Verification items for the finished model (mm, model axes). A direction names the side the tool comes from. Round coordinates to 2 decimals unless told otherwise and drop trailing zeros. Write each loop counter-clockwise with the first axis right and the second up, starting at its lowest first coordinate (ties: lowest second). Pieces come first, ordered by that corner, then holes. Notation, with made-up numbers: (-28, 26) - (-12, 26) arc R24 cw to (-12, 50) - close; hole circle Ø6 at (22, 5.25). An arc over 180 degrees is marked (long way). Answer as a JSON object with one key per item and string values.
```python
from build123d import *

# Parameters (mm, degrees)
SKETCH032_W     = 42
SKETCH032_H     = 42
PAD111_DEPTH    = 2
SKETCH165_W     = 24
SKETCH165_H     = 24
POCKET008_DEPTH = 1
SKETCH167_W     = 42
SKETCH167_H     = 42
SKETCH167_W_2   = 28
SKETCH167_H_2   = 28
POCKET009_DEPTH = 1
SKETCH300_R     = 1.1
POCKET045_DEPTH = 5


with BuildPart() as part:
    # Sketch032 → Pad111 (new body)
    with BuildSketch(Plane.XZ):
        Rectangle(SKETCH032_W, SKETCH032_H)
    extrude(amount=PAD111_DEPTH)

    # Sketch165 (on Face5 of Pad111) → Pocket008 (cut)
    with BuildSketch(Plane(origin=(0, 0, 0), x_dir=(1, 0, 0), z_dir=(0, 1, 0))):
        Rectangle(SKETCH165_W, SKETCH165_H)
    extrude(amount=-POCKET008_DEPTH, mode=Mode.SUBTRACT)

    # Sketch167 (on Face5 of Pocket008) → Pocket009 (cut)
    with BuildSketch(Plane.XZ.offset(2)):
        Rectangle(SKETCH167_W, SKETCH167_H)
        Rectangle(SKETCH167_W_2, SKETCH167_H_2, mode=Mode.SUBTRACT)
    extrude(amount=-POCKET009_DEPTH, mode=Mode.SUBTRACT)

    # Sketch300 (on Face16 of Pocket009) → Pocket045 (cut)
    with BuildSketch(Plane.XZ.offset(2)):
        with Locations((-10, 10)):
            Circle(SKETCH300_R)
        with Locations((10, -10)):
            Circle(SKETCH300_R)
    extrude(amount=-POCKET045_DEPTH, mode=Mode.SUBTRACT)


with BuildPart() as part_1:
    # Body012 placement: moved
    add(part.part.moved(Location((0, 7.5, 17.5))))


solid = part_1.part
```
Q1. Gauge pin test, flat ends, axial feed: P1, Ø6, axis at x = -7, z = 17.5, coming from the +Y side; P2, Ø0.8, axis at x = -4.5, y = 6, coming from the +Z side; P3, Ø0.8, axis at y = 6, z = 16.5, coming from the +X side; P4, Ø1.8, axis at x = -10, z = 27.5, coming from the -Y side. Record the tip position at first contact, or that the pin passes through.
Geometry check:
{"P1": "stops at y = 6.5", "P2": "stops at z = 31.5", "P3": "stops at x = 14", "P4": "passes through"}
Q2. Set-up check for faces 5 (the flat face through (0, 7, 29.5)), 6 (the flat face through (0, 6, 3.5)), 7 (the flat face through (0, 6, 31.5)): record each of +Z, -Z, +X, -X, +Y, -Y from which the full face is reachable in a straight line by a thin tool's end or side.
Geometry check:
{"face 5": "+Y", "face 6": "-Z, +X, -X, -Y", "face 7": "+Z, +X, -X, -Y"}
Q3. Material ranges on line 1 along X through (y, z) = (7.2, 16.5); line 2 along Z through (x, y) = (4, 7.2); line 3 along Z through (x, y) = (10, 5.8), recorded low to high. Write a range as [from, to].
Geometry check:
{"line 1": "x = [-21, -12], [12, 21]", "line 2": "z = [-3.5, 5.5], [29.5, 38.5]", "line 3": "z = [3.5, 6.4], [8.6, 31.5]"}
Q4. Section check D-D, the plane y = 6.1. Record the cut outline in (x, z), then the cut area to 3 significant figures.
Geometry check:
{"outline": "(-14, 3.5) - (14, 3.5) - (14, 31.5) - (-14, 31.5) - close; hole circle Ø2.2 at (-10, 27.5); hole circle Ø2.2 at (10, 7.5)", "area": "776 mm2"}
Q5. Release check for a two-part mould opening along X. For faces 1 (the flat face through (-21, 7, 17)), 2 (the flat face through (14, 6, 17)), 3 (the flat face through (0, 6.5, 32)), 4 (the flat face through (0, 6.5, 17)) record: released by +X, released by -X, zero draft, split by the parting line, or undercut.
Geometry check:
{"face 1": "released by -X", "face 2": "released by +X", "face 3": "zero draft", "face 4": "undercut"}
Q6. Section check B-B, the plane x = -10. Record the cut outline in (y, z).
Geometry check:
{"outline": "(5.5, 3.5) - (6.5, 3.5) - (6.5, -3.5) - (7.5, -3.5) - (7.5, 5.5) - (6.5, 5.5) - (6.5, 26.4) - (5.5, 26.4) - close; (5.5, 28.6) - (6.5, 28.6) - (6.5, 29.5) - (7.5, 29.5) - (7.5, 38.5) - (6.5, 38.5) - (6.5, 31.5) - (5.5, 31.5) - close"}
Q7. Section check C-C, the plane z = 10.5. Record the cut outline in (x, y).
Geometry check:
{"outline": "(-21, 6.5) - (-14, 6.5) - (-14, 5.5) - (14, 5.5) - (14, 6.5) - (21, 6.5) - (21, 7.5) - (12, 7.5) - (12, 6.5) - (-12, 6.5) - (-12, 7.5) - (-21, 7.5) - close"}
Q8. Section check A-A, the plane z = 27.5. Record the cut outline in (x, y), then the cut area to 3 significant figures.
Geometry check:
{"outline": "(-21, 6.5) - (-14, 6.5) - (-14, 5.5) - (-11.1, 5.5) - (-11.1, 6.5) - (-12, 6.5) - (-12, 7.5) - (-21, 7.5) - close; (-8.9, 5.5) - (14, 5.5) - (14, 6.5) - (21, 6.5) - (21, 7.5) - (12, 7.5) - (12, 6.5) - (-8.9, 6.5) - close", "area": "43.8 mm2"}
